```python
from build123d import *

# Parameters (mm, degrees)
SKETCH1_W                  = 16.3
SKETCH1_H                  = 3
BOSS_EXTRUDE1_DEPTH        = 2
SKETCH2_W                  = 2.9
SKETCH2_H                  = 3
BOSS_EXTRUDE2_DEPTH        = 1.5
SKETCH6_W                  = 0.8
SKETCH6_H                  = 1.5
BOSS_EXTRUDE4_DEPTH        = 3
F_1_4_1_4_DIAMETER_HOLE1_D = 1.4
CUT_EXTRUDE1_DEPTH         = 3
SKETCH9_W                  = 2.5
SKETCH9_H                  = 3
BOSS_EXTRUDE5_DEPTH        = 1.9
CUT_EXTRUDE2_DEPTH         = 10.520110293
CUT_EXTRUDE3_DEPTH         = 10
BOSS_EXTRUDE7_DEPTH        = 3


with BuildPart() as part:
    # Sketch1 → Boss-Extrude1 (new body)
    with BuildSketch(Plane(origin=(0, 0, 0), x_dir=(1, 0, 0), z_dir=(0, 1, 0))):
        Rectangle(SKETCH1_W, SKETCH1_H)
    extrude(amount=BOSS_EXTRUDE1_DEPTH)

    # Sketch2 → Boss-Extrude2 (add)
    with BuildSketch(Plane(origin=(0, 2, 0), x_dir=(1, 0, 0), z_dir=(0, 1, 0))):
        with Locations((5.9, 0)):
            Rectangle(SKETCH2_W, SKETCH2_H)
    extrude(amount=BOSS_EXTRUDE2_DEPTH)

    # Sketch6 → Boss-Extrude4 (add)
    with BuildSketch(Plane.XY.offset(1.5)):
        Polygon((4.45, 3.5), (2.8, 2), (4.45, 2), align=None)
        with Locations((7.75, 2.75)):
            Rectangle(SKETCH6_W, SKETCH6_H)
    extrude(amount=-BOSS_EXTRUDE4_DEPTH)

    # Ø1.4 (1.4) Diameter Hole1 (through all)
    with Locations(Plane.XY.offset(1.5)):
        with Locations((6.55, 2)):
            Hole(F_1_4_1_4_DIAMETER_HOLE1_D / 2)

    # Sketch8 → Cut-Extrude1 (cut)
    with BuildSketch(Plane.XY.offset(1.5)):
        Polygon((8.15, 0), (6.85, 0), (8.15, 1.3), align=None)
    extrude(amount=-CUT_EXTRUDE1_DEPTH, mode=Mode.SUBTRACT)

    # Sketch9 → Boss-Extrude5 (add)
    with BuildSketch(Plane(origin=(0, 2, 0), x_dir=(1, 0, 0), z_dir=(0, 1, 0))):
        with Locations((-6.9, 0)):
            Rectangle(SKETCH9_W, SKETCH9_H)
    extrude(amount=BOSS_EXTRUDE5_DEPTH)

    # Sketch10 → Cut-Extrude2 (cut, through all)
    with BuildSketch(Plane.XY.offset(1.5)):
        Polygon((-5.65, 3.9), (-5.65, 3.4), (-6.15, 3.9), align=None)
    extrude(amount=-CUT_EXTRUDE2_DEPTH, mode=Mode.SUBTRACT)

    # Sketch13 → Cut-Extrude3 (cut)
    with BuildSketch(Plane(origin=(0, 0, -1.5), x_dir=(-1, 0, 0), z_dir=(0, 0, -1))):
        Polygon((-8.15, 3.5), (-8.15, 2.5), (-7.15, 3.5), align=None)
    extrude(amount=-CUT_EXTRUDE3_DEPTH, mode=Mode.SUBTRACT)

    # Sketch14 → Boss-Extrude7 (add)
    with BuildSketch(Plane(origin=(0, 0, -1.5), x_dir=(-1, 0, 0), z_dir=(0, 0, -1))):
        with BuildLine():
            Line((-8.15, 1.3), (-7.15, 3.5))
            ThreePointArc((-7.15, 3.5), (-8.235707881, 2.666230855), (-8.15, 1.3))
        make_face()
    extrude(amount=-BOSS_EXTRUDE7_DEPTH)


solid = part.part
```
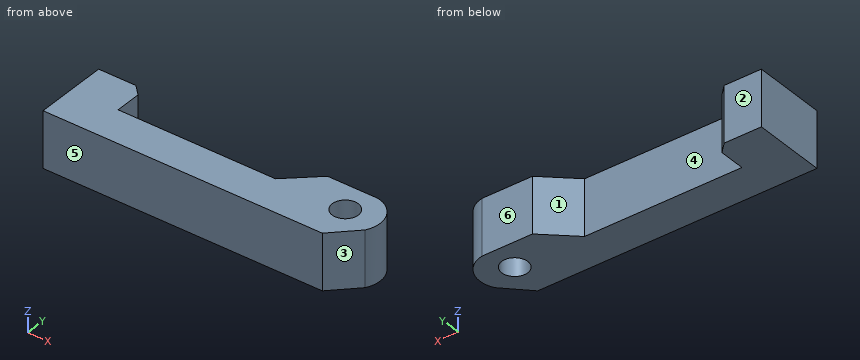
Could you check a few things on this model? Use its own coordinates, in mm. Face numbers are marked on the shaded views. A direction names the side the tool comes from. Give positions to 0.01 mm unless a question says otherwise; leave off trailing zeros. Write each loop counter-clockwise with the first axis right and the second up, starting at its lowest first coordinate (ties: lowest second). Pieces come first, ordered by that corner, then holes. Notation, with made-up numbers: (-2, -34) - (12, -34) arc R34 ccw to (12, 5) - close; hole circle Ø4 at (-32, 67). An arc over 180 degrees is marked (long way). One line per item, written item: value. Start each with the question number.
Item 1: I'm going to push a flat-ended pin straight in: pin 1 (0.9 mm diameter, centred on x = -2, z = -0.5, fed in from +Y). Where does the tip first touch, or does it pass through?
Item 2: Imagine slicing it at C-C, the plane y = 1.6. List the corners of the cut face in (x, z) for me.
Item 3: Imagine slicing it at A-A, the plane x = 6.55. List the corners of the cut face in (y, z) for me.
Item 4: Which directions (+Z, -Z, +X, -X, +Y, -Y) give clear straight access to the entire face, cutting with the end or side of a thin tool? Please do the marked faces 4, 5 and 6.
Item 5: If we mould it in two halves opening along X, with no side actions, what happens to the marked faces 1, 2 and 3? For each: +X half, -X half, draft (parallel to the pull), parting line (faces both ways), or undercut.
Item 6: Imagine slicing it at D-D, the plane y = 0.6. List the corners of the cut face in (x, z) for me.
Item 7: Please list where these lines run through material, in increasing order: line 1 (Y direction, x = 6.55, z = -0.35); line 2 (X direction, y = 2.4, z = -0.95); line 3 (X direction, y = 2.55, z = 0.5) (3 decimals). Write a range as from..to.
Item 8: Imagine slicing it at B-B, the plane z = -0.65. List the corners of the cut face in (x, y) for me, and give its area (3 significant figures).
Geometry says:
1. pin 1: y = 2
2. outline: (-8.15, -1.5) - (5.98, -1.5) - (5.98, 1.5) - (-8.15, 1.5) - close; (7.12, -1.5) - (8.29, -1.5) - (8.29, 1.5) - (7.12, 1.5) - close
3. outline: (0, -1.5) - (1.3, -1.5) - (1.3, 1.5) - (0, 1.5) - close; (2.7, -1.5) - (3.5, -1.5) - (3.5, 1.5) - (2.7, 1.5) - close
4. face 4: +Z, -Z, +Y
4. face 5: +Z, -Z, +X, -X, -Y
4. face 6: +Z, -Z, +X, +Y
5. face 1: undercut
5. face 2: draft
5. face 3: +X half
6. outline: (-8.15, -1.5) - (7.45, -1.5) - (7.45, 1.5) - (-8.15, 1.5) - close
7. line 1: 0..1.3, 2.7..3.5
7. line 2: -8.15..-5.65, 3.24..5.98, 7.12..8.33
7. line 3: -8.15..-5.65, 3.405..6.117, 6.983..8.283
8. outline: (-8.15, 0) - (6.85, 0) - (8.15, 1.3) arc R1.46 ccw to (7.15, 3.5) - (4.45, 3.5) - (2.8, 2) - (-5.65, 2) - (-5.65, 3.4) - (-6.15, 3.9) - (-8.15, 3.9) - close; hole circle Ø1.4 at (6.55, 2)
8. area: 41.6 mm^2
